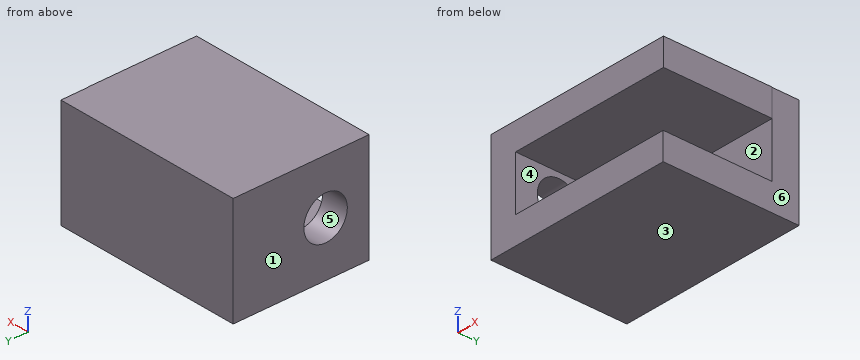
```python
from build123d import *

# Parameters (mm, degrees)
SKETCH1_W           = 19.05
SKETCH1_H           = 12.7
BOSS_EXTRUDE1_DEPTH = 3.175
SKETCH3_W           = 19.014556256
SKETCH3_H           = 12.7
BOSS_EXTRUDE2_DEPTH = 3.175
SKETCH5_W           = 12.7
SKETCH5_H           = 15.875
BOSS_EXTRUDE4_DEPTH = 3.175
SKETCH6_R           = 2.54
CUT_EXTRUDE1_DEPTH  = 23.225
SKETCH4_W           = 19.014556256
SKETCH4_H           = 3.175
BOSS_EXTRUDE5_DEPTH = 12.7


with BuildPart() as part:
    # Sketch1 → Boss-Extrude1 (new body)
    with BuildSketch(Plane.XY):
        with Locations((9.525, 6.35)):
            Rectangle(SKETCH1_W, SKETCH1_H)
    extrude(amount=BOSS_EXTRUDE1_DEPTH)

    # Sketch3 → Boss-Extrude2 (add)
    with BuildSketch(Plane(origin=(0, 12.7, 0), x_dir=(1, 0, 0), z_dir=(0, 1, 0))):
        with Locations((9.507278128, 3.175)):
            Rectangle(SKETCH3_W, SKETCH3_H)
    extrude(amount=BOSS_EXTRUDE2_DEPTH)

    # Sketch5 → Boss-Extrude4 (add)
    with BuildSketch(Plane.ZY):
        with Locations((-3.175, 7.9375)):
            Rectangle(SKETCH5_W, SKETCH5_H)
    extrude(amount=BOSS_EXTRUDE4_DEPTH)

    # Sketch6 → Cut-Extrude1 (cut, through all)
    with BuildSketch(Plane.ZY.offset(3.175)):
        with Locations((-3.175, 5.08)):
            Circle(SKETCH6_R)
    extrude(amount=-CUT_EXTRUDE1_DEPTH, mode=Mode.SUBTRACT)

    # Sketch4 → Boss-Extrude5 (add)
    with BuildSketch(Plane.XZ.offset(-12.7)):
        with Locations((9.507278128, -7.9375)):
            Rectangle(SKETCH4_W, SKETCH4_H)
    extrude(amount=BOSS_EXTRUDE5_DEPTH)


solid = part.part
```
Geometry check sheet. Reference: the model listing, model coordinates, mm. Face numbers are marked on the shaded views. A direction names the side the tool comes from. Coordinates: 2 decimals unless noted, no trailing zeros. Loops run counter-clockwise (first coordinate to the right, second up) from the corner with the lowest first, then second, coordinate; pieces in that order, holes last.
Item 1: Sectioned sample at A-A, the plane y = 5.08. Record the boundary of the cut face in (x, z) (3 decimals).
Item 2: Sectioned sample at C-C, the plane x = 12.75. Record the boundary of the cut face in (y, z) (3 decimals), then the cut area to 3 significant figures.
Item 3: Access from +Z, -Z, +X, -X, +Y, -Y to the whole of each face (thin tool, end or side, straight path). Record for the marked faces 4, 5 and 6.
Item 4: Thickness scan on line 1 (Z direction, x = 1.75, y = 9.5) (3 decimals); line 2 (X direction, y = 8, z = -0.25) (3 decimals); line 3 (Y direction, x = 8, z = -2.5) (3 decimals). Record the ranges inside material, lowest first.
Item 5: Sectioned sample at D-D, the plane y = 1.75. Record the boundary of the cut face in (x, z) (3 decimals).
Item 6: Sectioned sample at B-B, the plane z = -2. Record the boundary of the cut face in (x, y) (3 decimals), then the cut area to 3 significant figures.
Item 7: Release check for a two-part mould opening along Z. For the marked faces 1, 2 and 3 record: released by +Z, released by -Z, zero draft, split by the parting line, or undercut.
Check result:
1. outline: (-3.175, -9.525) - (19.015, -9.525) - (19.015, -6.35) - (0, -6.35) - (0, -5.715) - (-3.175, -5.715) - close; (-3.175, -0.635) - (0, -0.635) - (0, 0) - (19.05, 0) - (19.05, 3.175) - (-3.175, 3.175) - close
2. outline: (0, -9.525) - (15.875, -9.525) - (15.875, 3.175) - (0, 3.175) - (0, 0) - (12.7, 0) - (12.7, -6.35) - (0, -6.35) - close
2. area: 121 mm2
3. face 4: +X, -Y
3. face 5: +X, -X
3. face 6: -Z, +X, +Y
4. line 1: z = -9.525 to -6.35, 0 to 3.175
4. line 2: x = -3.175 to 0
4. line 3: y = 12.7 to 15.875
5. outline: (-3.175, -9.525) - (19.015, -9.525) - (19.015, -6.35) - (0, -6.35) - (0, 0) - (19.05, 0) - (19.05, 3.175) - (-3.175, 3.175) - close
6. outline: (-3.175, 0) - (0, 0) - (0, 2.828) - (-3.175, 2.828) - close; (-3.175, 7.332) - (0, 7.332) - (0, 12.7) - (19.015, 12.7) - (19.015, 15.875) - (-3.175, 15.875) - close
6. area: 96.5 mm2
7. face 1: zero draft
7. face 2: undercut
7. face 3: released by -Z
